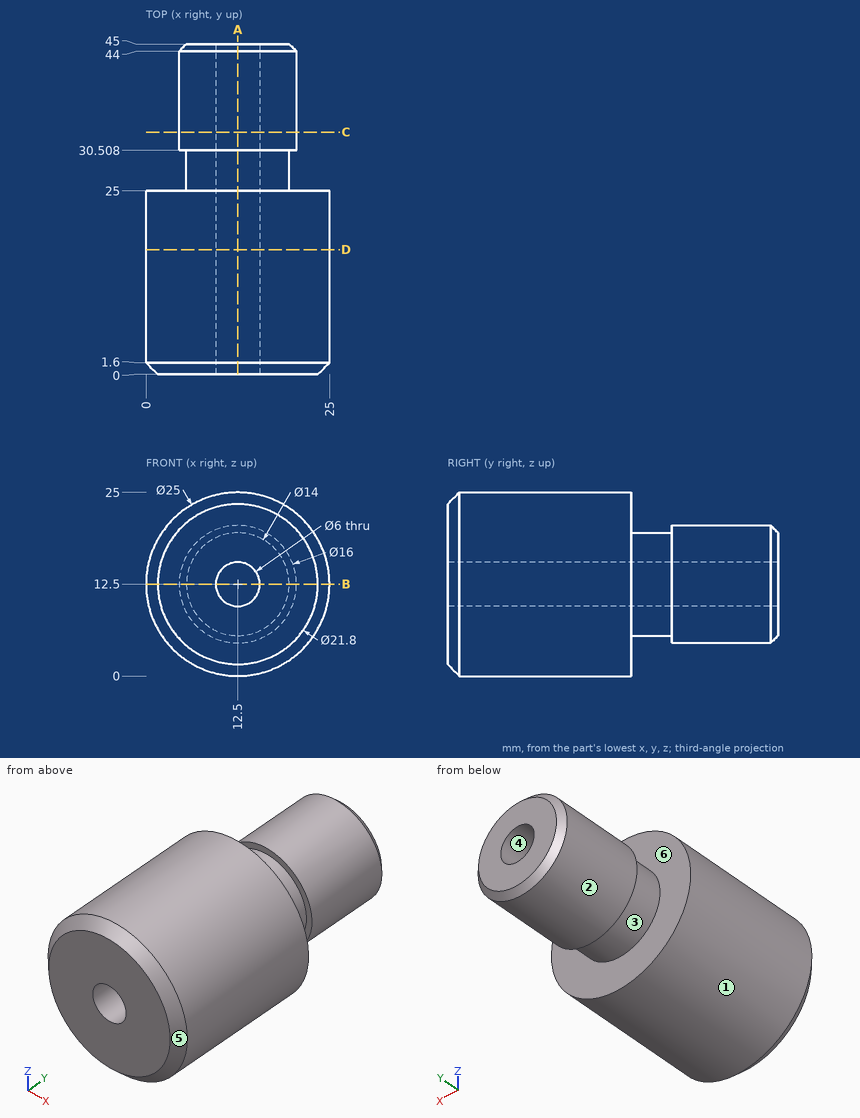
Drawing for the job (mm, zero at the part's lowest x, y, z). A direction names the side the tool comes from. Give positions to 0.01 mm unless a question says otherwise; leave off trailing zeros. Order: outer loops, then holes, each group sorted by start corner. A loop starts at its lowest first (then second) coordinate and runs counter-clockwise, first axis right, second up. Notation, with made-up numbers: M -3,82.25 L 22,82.25 A31 cw 22,114.25 Z; hole C -1.5,36.25 d11. An arc over 180 degrees is marked long. Write item = value, one per line. Start each with the question number.
(1) Slice it at C-C on y = 33. Write the cut outline in (x, z).
(2) Slice it at B-B on z = 12.5. Write the cut outline in (x, y).
(3) Probe L1, parallel to X at y = 14, z = 12.5; L2, parallel to Z at x = 12.5, y = 32. List the from-to ranges inside material, lowest first. Write a range as [from, to].
(4) Slice it at D-D on y = 17. Write the cut outline in (x, z).
(5) Slice it at A-A on x = 12.5. Write the cut outline in (y, z).
(6) Pin check, flat tips, straight feed: pin 1 Ø5 at (y, z) = (30, 8) entering from +X; pin 2 Ø1.5 at (y, z) = (37.5, 10.5) entering from +X; pin 3 Ø1 at (y, z) = (23, 4.5) entering from +X. Stop position of each tip, or through.
(7) Which spindle directions (+Z, -Z, +X, -X, +Y, -Y) get a long thin tool onto all of the face, cutting with end or side? Do the marked faces 1, 2 and 3. Say none if no direction does.
(8) Two-plate mould, pull along X, no slides. Class the marked faces 4, 5 and 6: released by +X, released by -X, zero draft, split by the parting line, or undercut.
Responses:
q1.outline = C 12.5,12.5 d16; hole C 12.5,12.5 d6
q2.outline = M 0,1.6 L 1.6,0 L 9.5,0 L 9.5,45 L 5.5,45 L 4.5,44 L 4.5,30.51 L 5.5,30.51 L 5.5,25 L 0,25 Z; M 15.5,0 L 23.4,0 L 25,1.6 L 25,25 L 19.5,25 L 19.5,30.51 L 20.5,30.51 L 20.5,44 L 19.5,45 L 15.5,45 Z
q3.L1 = [0, 9.5], [15.5, 25]
q3.L2 = [4.5, 9.5], [15.5, 20.5]
q4.outline = C 12.5,12.5 d25; hole C 12.5,12.5 d6
q5.outline = M 0,1.6 L 1.6,0 L 25,0 L 25,5.5 L 30.51,5.5 L 30.51,4.5 L 44,4.5 L 45,5.5 L 45,9.5 L 0,9.5 Z; M 0,15.5 L 45,15.5 L 45,19.5 L 44,20.5 L 30.51,20.5 L 30.51,19.5 L 25,19.5 L 25,25 L 1.6,25 L 0,23.4 Z
q6.pin_1 = 20.23
q6.pin_2 = 20.4
q6.pin_3 = 22.5
q7.face_1 = +Y, -Y
q7.face_2 = +Y
q7.face_3 = none
q8.face_4 = undercut
q8.face_5 = split by the parting line
q8.face_6 = zero draft
